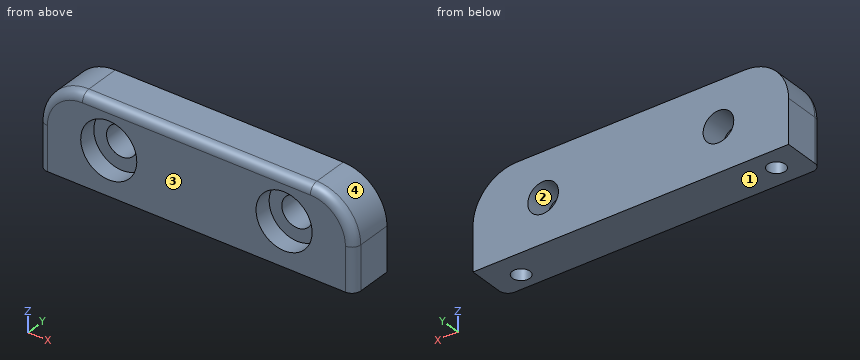
from build123d import *

# Parameters (mm, degrees)
SKETCH_1_W             = 36
SKETCH_1_H             = 5
EXTRUDE_376_DEPTH      = 5
SKETCH_4_R             = 1
I2C_DEPTH              = 9
SKETCH_5_R             = 1.75
CUT_EXTRUDE_974_DEPTH  = 20.339079606
SKETCH_6_R             = 3.2
CUT_EXTRUDE_1213_DEPTH = 2
FILLET_1_R             = 5
FILLET_2_R             = 1


with BuildPart() as part:
    # Эскиз1 → Extrude 376 (new, symmetric)
    with BuildSketch(Plane.XY):
        Rectangle(SKETCH_1_W, SKETCH_1_H)
    extrude(amount=EXTRUDE_376_DEPTH, both=True)

    # Эскиз4 → i2c (cut)
    with BuildSketch(Plane(origin=(0, 0, -5), x_dir=(-1, 0, 0), z_dir=(0, 0, -1))):
        with Locations((-14.75, -0.5)):
            Circle(SKETCH_4_R)
        with Locations((14.75, 0)):
            Circle(SKETCH_4_R)
    extrude(amount=-I2C_DEPTH, mode=Mode.SUBTRACT)

    # Эскиз5 → Cut-Extrude 974 (cut, through all)
    with BuildSketch(Plane(origin=(0, 2.5, 0), x_dir=(1, 0, 0), z_dir=(0, 1, 0))):
        with Locations(Location((-10, 0, 0), (0, 0, 270))):
            Circle(SKETCH_5_R)
        with Locations(Location((10, 0, 0), (0, 0, 270))):
            Circle(SKETCH_5_R)
    extrude(amount=-CUT_EXTRUDE_974_DEPTH, mode=Mode.SUBTRACT)

    # Эскиз6 → Cut-Extrude 1213 (cut)
    with BuildSketch(Plane(origin=(0, -2.5, 0), x_dir=(1, 0, 0), z_dir=(0, 1, 0))):
        with Locations(Location((-10, 0, 0), (0, 0, 90))):
            Circle(SKETCH_6_R)
        with Locations(Location((10, 0, 0), (0, 0, 90))):
            Circle(SKETCH_6_R)
    extrude(amount=CUT_EXTRUDE_1213_DEPTH, mode=Mode.SUBTRACT)

    # Скругление1
    fillet_1_edges = [part.edges().sort_by_distance(p)[0] for p in [
        (18, 0, 5),
        (-18, 0, 5),
    ]]
    fillet(fillet_1_edges, radius=FILLET_1_R)

    # Скругление2
    fillet_2_edges = [part.edges().sort_by_distance(p)[0] for p in [
        (0, -2.5, 5),
        (18, -2.5, -2.5),
        (-18, -2.5, -2.5),
        (16.535533906, -2.5, 3.535533906),
        (-16.535533906, -2.5, 3.535533906),
    ]]
    fillet(fillet_2_edges, radius=FILLET_2_R)


solid = part.part
Geometry check sheet. Reference: the model listing, model coordinates, mm. Face numbers are marked on the shaded views. Round coordinates to 2 decimals unless told otherwise and drop trailing zeros. Write each loop counter-clockwise with the first axis right and the second up, starting at its lowest first coordinate (ties: lowest second). Pieces come first, ordered by that corner, then holes. Notation, with made-up numbers: (29.25, -31) -> (74.25, -31) arc R20 ccw to (74.25, -27) -> close; hole circle Ø9 at (68.5, 36.25). An arc over 180 degrees is marked (long way). One line per item, written item: value. Start each with the question number.
(1) Go/stop test with flat-tipped pins: pin 1 Ø5.5 at (x, z) = (10, 0) entering from -Y; pin 2 Ø1.6 at (x, y) = (-14.75, 0) entering from -Z; pin 3 Ø1.6 at (x, y) = (14.75, -0.5) entering from +Z. Record where each tip stops, or that it passes through.
(2) Cross-section at B-B, the plane z = -1. Record the cut outline in (x, y), and give its area (3 significant figures).
(3) Cross-section at C-C, the plane x = 10. Record the cut outline in (y, z), and give its area (3 significant figures).
(4) Scan lines: line 1 (X direction, y = -0.05, z = 3.5); line 2 (X direction, y = 1.1, z = -0.5); line 3 (Y direction, x = -14.75, z = -3). Record each from-to range of solid material in increasing order. Write a range as [from, to].
(5) Draft check along Z on the marked faces 1, 2, 3 and 4. Enter one of: +Z half, -Z half, draft (parallel to the pull), parting line (faces both ways), or undercut.
(6) Cross-section at A-A, the plane y = 1.6. Record the cut outline in (x, z), and give its area (3 significant figures).
(7) Cross-section at D-D, the plane z = 2.5. Give the number of separate pieces and of enclosed holes in the cut face, and give its area (3 significant figures).
Answer:
1. pin 1: y = -0.5
1. pin 2: z = 4
1. pin 3: z = 4.91
2. outline: (-18, -1.5) arc R1 ccw to (-17, -2.5) -> (-13.04, -2.5) -> (-13.04, -0.5) -> (-11.44, -0.5) -> (-11.44, 2.5) -> (-18, 2.5) -> close; (-8.56, -0.5) -> (-6.96, -0.5) -> (-6.96, -2.5) -> (6.96, -2.5) -> (6.96, -0.5) -> (8.56, -0.5) -> (8.56, 2.5) -> (-8.56, 2.5) -> close; (11.44, -0.5) -> (13.04, -0.5) -> (13.04, -2.5) -> (17, -2.5) arc R1 ccw to (18, -1.5) -> (18, 2.5) -> (11.44, 2.5) -> close; hole circle Ø2 at (-14.75, 0); hole circle Ø2 at (14.75, -0.5)
2. area: 132 mm²
3. outline: (-2.5, -5) -> (2.5, -5) -> (2.5, -1.75) -> (-0.5, -1.75) -> (-0.5, -3.2) -> (-2.5, -3.2) -> close; (-2.5, 3.2) -> (-0.5, 3.2) -> (-0.5, 1.75) -> (2.5, 1.75) -> (2.5, 5) -> (-1.5, 5) arc R1 ccw to (-2.5, 4) -> close
3. area: 26.5 mm²
4. line 1: [-16.57, -15.75], [-13.75, 13.86], [15.64, 16.57]
4. line 2: [-18, -11.68], [-8.32, 8.32], [11.68, 18]
4. line 3: [-2.5, -1], [1, 2.5]
5. face 1: -Z half
5. face 2: undercut
5. face 3: draft
5. face 4: +Z half
6. outline: (-18, -5) -> (18, -5) -> (18, 0) arc R5 ccw to (13, 5) -> (-13, 5) arc R5 ccw to (-18, 0) -> close; hole circle Ø3.5 at (-10, 0); hole circle Ø3.5 at (10, 0)
6. area: 330 mm²
7. separate pieces: 1
7. enclosed holes: 2
7. area: 151 mm²
